Design review of the part built by this model. Coordinates are the model's own, in mm. A direction names the side the tool comes from. Round coordinates to 2 decimals unless told otherwise and drop trailing zeros. Write each loop counter-clockwise with the first axis right and the second up, starting at its lowest first coordinate (ties: lowest second). Pieces come first, ordered by that corner, then holes. Notation, with made-up numbers: (-38, 55.25) -> (4, 55.25) arc R11 cw to (4, 75.25) -> close; hole circle Ø10 at (14.25, 69). An arc over 180 degrees is marked (long way). One line per question, with ' | ' between items. Start each with the question number.
1) For probe 1 along Z at (x, y) = (-3.5, -3); probe 2 along X at (y, z) = (-0.75, 46); probe 3 along X at (y, z) = (-2, 69), list the stretches that pass through material, from the lowest coordinate up.
2) Consider section D-D (z = 68). Give the boundary of the cut face in (x, y) (3 decimals).
3) Consider section B-B (z = 44.5). Give the boundary of the cut face in (x, y), then the cut area to 3 significant figures.
4) Consider section A-A (x = -26.5). Give the boundary of the cut face in (y, z), then the cut area to 3 significant figures.
5) Mouldability with a two-part tool opening along Z and no side actions: class faces 1 (the flat face through (-17.42, 5.06, 10.42)), 2 (the flat face through (-1.25, 5.06, 5.75)), 3 (the flat face through (-22.226, -5.062, 74.451)) as +Z half, -Z half, draft (parallel to the pull), parting line (faces both ways), or undercut.
6) Consider section C-C (y = -1.75). Give the boundary of the cut face in (x, z), then the cut area to 3 significant figures.
7) For faces 4 (the flat face through (-1.25, 5.06, 69.78)), 5 (the flat face through (-32.793, 0, 37)), 6 (the flat face through (-17.91, 5.06, 65.27)), list the 3-axis set-ups (+Z, -Z, +X, -X, +Y, -Y) from which the entire face can be reached by the end or side of a thin tool; tool diameter is ignored.
8) Insertion check: pin 1 Ø7.5 at (x, y) = (-6.17, 0.11) entering from -Z; pin 2 Ø1 at (y, z) = (-1.5, 14.5) entering from +X. Each pin has a flat end and moves straight along its axis. Give the tip position at first contact, or say it passes through.
```python
from build123d import *

# Parameters (mm, degrees)
F1_DEPTH = 6.35
F3_D     = 6.35
F4_SIZE  = 2.54
F5_SIZE  = 2.54
F6_SIZE  = 2.53999


# Not quite as in the source:
# - a fillet or chamfer is up to 0.001 mm smaller than in the source, because OpenCascade refuses the exact size


with BuildPart() as f1:
    # F0 (on Front) → F1 (new body, symmetric)
    with BuildSketch(Plane.XZ):
        Polygon((-45.0841039419, 0), (0, 0), (0, 11.6680786014), (-32.7930003405, 11.6680786014), (-32.7930003405, 64.019061625), (0, 64.019061625), (0, 75.703188777), (-45.0841039419, 75.703188777), align=None)
    extrude(amount=F1_DEPTH, both=True)

    # F3 (through all)
    with Locations(Plane(origin=(0, 0, 0), x_dir=(1, 0, 0), z_dir=(0, 0, -1))):
        with Locations((-6.1689345166, -0.1147333004)):
            Hole(F3_D / 2)

    # F4
    f4_edges = [f1.edges().sort_by_distance(p)[0] for p in [
        (-22.542052, -6.35, 75.703189),
        (-22.542052, 6.35, 75.703189),
        (-16.3965, -6.35, 64.019062),
        (0, -6.35, 69.861125),
        (0, 6.35, 69.861125),
        (-16.3965, 6.35, 64.019062),
    ]]
    chamfer(f4_edges, length=F4_SIZE)

    # F5
    f5_edges = [f1.edges().sort_by_distance(p)[0] for p in [
        (-22.542052, 6.35, 0),
        (0, -6.35, 5.834039),
        (-22.542052, -6.35, 0),
        (-16.3965, -6.35, 11.668079),
        (0, 6.35, 5.834039),
        (-16.3965, 6.35, 11.668079),
    ]]
    chamfer(f5_edges, length=F5_SIZE)

    # F6 (size 2.54 in the source; OpenCascade refuses exactly that, so slightly less here)
    f6_edges = [f1.edges().sort_by_distance(p)[0] for p in [
        (-45.084104, 6.35, 37.851594),
        (-32.793, -6.35, 37.84357),
        (-32.793, 6.35, 37.84357),
        (-45.084104, -6.35, 37.851594),
    ]]
    chamfer(f6_edges, length=F6_SIZE)


solid = f1.part
```
From the geometry:
1) probe 1: z = 0 to 11.67, 64.02 to 75.7 | probe 2: x = -45.08 to -32.79 | probe 3: x = -45.08 to -8.54, -3.8 to 0
2) outline: (-45.084, -3.81) -> (-42.544, -6.35) -> (-2.54, -6.35) -> (0, -3.81) -> (0, 3.81) -> (-2.54, 6.35) -> (-42.544, 6.35) -> (-45.084, 3.81) -> close; hole circle Ø6.35 at (-6.169, 0.115)
3) outline: (-45.08, -3.81) -> (-42.54, -6.35) -> (-35.33, -6.35) -> (-32.79, -3.81) -> (-32.79, 3.81) -> (-35.33, 6.35) -> (-42.54, 6.35) -> (-45.08, 3.81) -> close | area: 143 mm2
4) outline: (-6.35, 2.54) -> (-3.81, 0) -> (3.81, 0) -> (6.35, 2.54) -> (6.35, 9.13) -> (3.81, 11.67) -> (-3.81, 11.67) -> (-6.35, 9.13) -> close; (-6.35, 66.56) -> (-3.81, 64.02) -> (3.81, 64.02) -> (6.35, 66.56) -> (6.35, 73.16) -> (3.81, 75.7) -> (-3.81, 75.7) -> (-6.35, 73.16) -> close | area: 271 mm2
5) face 1: undercut | face 2: draft | face 3: +Z half
6) outline: (-45.08, 0) -> (-8.74, 0) -> (-8.74, 11.67) -> (-32.79, 11.67) -> (-32.79, 64.02) -> (-8.74, 64.02) -> (-8.74, 75.7) -> (-45.08, 75.7) -> close; (-3.6, 0) -> (0, 0) -> (0, 11.67) -> (-3.6, 11.67) -> close; (-3.6, 64.02) -> (0, 64.02) -> (0, 75.7) -> (-3.6, 75.7) -> close | area: 1,580 mm2
7) face 4: +Z, -Z, +X, +Y | face 5: +X, +Y, -Y | face 6: +X, +Y
8) pin 1: stops at z = 0 | pin 2: stops at x = -32.79
